The model under review builds one solid part; all positions refer to its coordinate system, in mm. Face numbers are marked on the shaded views. A direction names the side the tool comes from. Round coordinates to 2 decimals unless told otherwise and drop trailing zeros. Write each loop counter-clockwise with the first axis right and the second up, starting at its lowest first coordinate (ties: lowest second). Pieces come first, ordered by that corner, then holes. Notation, with made-up numbers: M -38.75,-13 L 2.25,-13 A16 cw 2.25,-3 Z; hole C -20.5,32 d3. An arc over 180 degrees is marked long. One line per item, written item: value. Start each with the question number.
1) Tool access review of the marked faces 1 and 2: name each direction out of +Z, -Z, +X, -X, +Y, -Y from which nothing blocks a thin tool from reaching the whole face with its end or side.
2) Take a section at B-B, the plane z = 15. Write out the cut boundary in (x, y), and give its area (3 significant figures).
3) Take a section at D-D, the plane y = 9.5. Write out the cut boundary in (x, z).
4) Mouldability with a two-part tool opening along Y and no side actions: class the marked faces 3, 4 and 5 as +Y half, -Y half, draft (parallel to the pull), parting line (faces both ways), or undercut.
5) Take a section at C-C, the plane x = 15. Write out the cut boundary in (y, z).
6) Wall thickness on probe 1 along Y at (x, z) = (5, 26); probe 2 along Z at (x, y) = (-5, 1.5): over which ranges is each line inside the solid? List them lowest first.
7) Take a section at A-A, the plane y = 5. Write out the cut boundary in (x, z).
8) For P1, Ø4, axis at y = 5.5, z = 10, coming from the +X side; P2, Ø13, axis at x = 6, z = 14.5, coming from the +Y side; P3, Ø5, axis at y = 3.79, z = 7, coming from the -X side; P4, Ø1, axis at x = -1, z = 25, coming from the +Y side, all flat-tipped, find the tip position at first contact; note any pin that passes through.
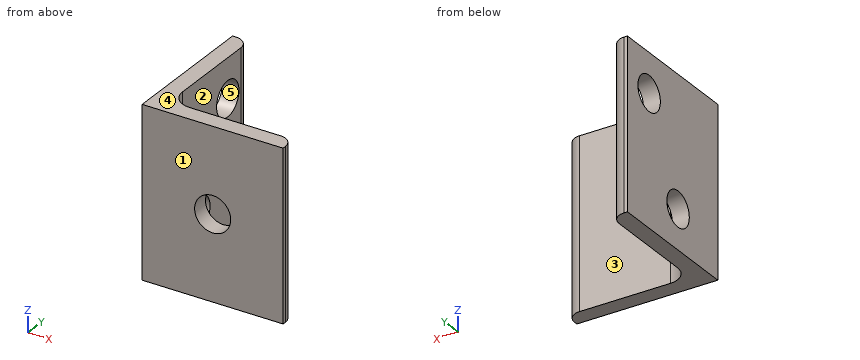
Autodesk Inventor part; units mm, degrees
ref_plane "Počáteční rovina" through (0, 0, 0) normal (0, 0, 1) x (1, 0, 0)
ref_plane "Koncová rovina" through (0, 0, 30) normal (0, 0, 1) x (1, 0, 0)
ref_plane "YZ Plane" through (0, 0, 0) normal (1, 0, 0) x (0, 1, 0)
ref_plane "Počáteční rovina" through (0, 0, 0) normal (0, 0, 1) x (1, 0, 0)
ref_plane "Koncová rovina" through (0, 0, 30) normal (0, 0, 1) x (1, 0, 0)
sketch "Náčrt2" plane through (0, 0, 0) normal (0, 0, 1) x (1, 0, 0)
  line L0 (-4.2069, -0.7069) -> (-4.2069, 15.3931)
  line L1 (-7.2069, 17.7931) -> (-6.6069, 17.7931)
  line L2 (-7.2069, -7.2069) -> (-7.2069, 17.7931)
  line L3 (-7.2069, -7.2069) -> (17.7931, -7.2069)
  line L4 (17.7931, -6.6069) -> (17.7931, -7.2069)
  line L5 (-0.7069, -4.2069) -> (15.3931, -4.2069)
  arc A0 (-4.2069, -0.7069) -> (-0.7069, -4.2069) centre (-0.7069, -0.7069) ccw
  arc A1 (-4.2069, 15.3931) -> (-6.6069, 17.7931) centre (-6.6069, 15.3931) ccw
  arc A2 (17.7931, -6.6069) -> (15.3931, -4.2069) centre (15.3931, -6.6069) ccw
  line L6 (0, 23.3895) -> (0, -12.3063) construction
  line L7 (-12.3063, 0) -> (23.3895, 0) construction
  point P0 (-4.2069, -4.2069)
  point P1 (-4.2069, 17.7931)
  point P2 (17.7931, -4.2069)
  dimension "d4" = 25
  dimension "d6" = 25
  dimension "d8" = 3
  dimension "d10" = 3
  dimension "d17" = 3.5
  dimension "d18" = 2.4
  dimension "d19" = 7.2069
  dimension "d20" = 7.2069
extrude "Těleso" add sketch "Náčrt2" along normal up to surface (30 mm away) from surface at 0
sketch "Sketch3" plane through (0, 0, 0) normal (0, 0, 1) x (1, 0, 0)
  line L0 (0, 0) -> (10, 0)
ref_plane "Work Plane10" through (0, 0, 0) normal (0, -1, 0) x (1, 0, 0)
sketch "Sketch4" plane through (0, 0, 0) normal (0, -1, 0) x (1, 0, 0)
  line L0 (-2, 0) -> (12, 0)
  line L1 (-2, 30) -> (12, 30)
  dimension "d24" = 30
sketch "Sketch5" plane through (-7.2069, 17.7931, 0) normal (-1, 0, 0) x (0, 0, 1)
  circle A0 centre (22.9996, -6) radius 3.1
  circle A1 centre (6.9996, -14) radius 3.1
  line L0 (0, -2.4) -> (0, -18.5)
  line L1 (30, -18.5) -> (0, -18.5)
  line L2 (30, -2.4) -> (30, -18.5)
  line L3 (30, -2.4) -> (0, -2.4)
  point P0 (0, -17.7931)
extrude "Extrusion2" cut sketch "Sketch5" against normal blind 10 contours A0 | A1
sketch "Sketch6" plane through (-7.2069, -7.2069, 0) normal (0, -1, 0) x (1, 0, 0)
  line L0 (22.6, 30) -> (25, 30) construction
  line L1 (0, 0) -> (0, 30) construction
  line L2 (25, 30) -> (0, 0) construction
  line L3 (22.6, 0) -> (25, 0) construction
  line L4 (25, 0) -> (0, 30) construction
  circle A0 centre (12.5, 15) radius 3.2
  point P0 (7.2069, 0)
  dimension "d27" = 6.4
extrude "Extrusion3" cut sketch "Sketch6" against normal blind 10
equation "\"d4\" = b"
equation "\"d6\" = b"
equation "\"d17\" = R"
equation "\"d18\" = R1"
equation "\"d19\" = ex"
equation "\"d20\" = d19"
equation "\"d11\" = G_L"
equation "\"b\" = 25"
equation "\"ParT\" = 3"
equation "\"R\" = 3.5"
equation "\"R1\" = 2.4"
equation "\"G_L\" = d24"
equation "\"G_OFFSET_START\" = 0"
equation "\"G_OFFSET_END\" = 0"
properties part number "BS 4848 - 25x25x3-30" material "Steel, Mild"
Checked values:
1. face 1: +Z, -Z, +X, -X, -Y
1. face 2: +Z, -Z, +X, +Y
2. outline: M -7.21,-7.21 L 2.09,-7.21 L 2.09,-4.21 L -0.71,-4.21 A3.5 cw -4.21,-0.71 L -4.21,15.39 A2.4 ccw -6.61,17.79 L -7.21,17.79 Z; M 8.49,-7.21 L 17.79,-7.21 L 17.79,-6.61 A2.4 ccw 15.39,-4.21 L 8.49,-4.21 Z
2. area: 122 mm2
3. outline: M -7.21,0 L -4.21,0 L -4.21,20.91 L -7.21,20.91 Z; M -7.21,25.09 L -4.21,25.09 L -4.21,30 L -7.21,30 Z
4. face 3: +Y half
4. face 4: draft
4. face 5: undercut
5. outline: M -7.21,0 L -4.21,0 L -4.21,30 L -7.21,30 Z
6. probe 1: y = -7.21 to -4.21
6. probe 2: z = 0 to 4.91, 9.09 to 30
7. outline: M -7.21,0 L -4.21,0 L -4.21,4.14 L -7.21,4.14 Z; M -7.21,9.86 L -4.21,9.86 L -4.21,30 L -7.21,30 Z
8. P1: stops at x = -4.21
8. P2: stops at y = -4.21
8. P3: passes through
8. P4: stops at y = -4.12
